from build123d import *

# Parameters (mm, degrees)
ESTRUSIONE_ESTRUSIONE1_DEPTH = 5
SCHIZZO2_W                   = 16
SCHIZZO2_H                   = 5
ESTRUSIONE_ESTRUSIONE2_DEPTH = 20
TAGLIO_ESTRUSIONE1_REACH     = 42.62
SCHIZZO3_R                   = 3.25


with BuildPart() as part:
    # Schizzo1 → Estrusione-Estrusione1 (new body)
    with BuildSketch(Plane.XY):
        Polygon((-16, 0), (0, 0), (0, -10), (20, -10), (20, -30), (4, -30), (-16, -9.295201316), align=None)
        with BuildLine():
            Line((16, -22.25), (6, -22.25))
            ThreePointArc((6, -22.25), (4.25, -24), (6, -25.75))
            Line((6, -25.75), (16, -25.75))
            ThreePointArc((16, -25.75), (17.75, -24), (16, -22.25))
        make_face(mode=Mode.SUBTRACT)
        with BuildLine():
            Line((16, -12.75), (6, -12.75))
            ThreePointArc((6, -12.75), (4.25, -14.5), (6, -16.25))
            Line((6, -16.25), (16, -16.25))
            ThreePointArc((16, -16.25), (17.75, -14.5), (16, -12.75))
        make_face(mode=Mode.SUBTRACT)
    extrude(amount=ESTRUSIONE_ESTRUSIONE1_DEPTH)

    # Schizzo2 → Estrusione-Estrusione2 (add)
    with BuildSketch(Plane.XY.offset(5)):
        with Locations((-8, -2.5)):
            Rectangle(SCHIZZO2_W, SCHIZZO2_H)
    extrude(amount=ESTRUSIONE_ESTRUSIONE2_DEPTH)

    # Schizzo3 → Taglio-Estrusione1 (cut, up to next)
    with BuildSketch(Plane.XZ.offset(5), mode=Mode.PRIVATE) as taglio_estrusione1_sk1:
        with Locations((-8, 17.5)):
            Circle(SCHIZZO3_R)
    taglio_estrusione1_tool1 = extrude(taglio_estrusione1_sk1.sketch, amount=-TAGLIO_ESTRUSIONE1_REACH, mode=Mode.PRIVATE) & part.part
    add(taglio_estrusione1_tool1.solids().sort_by_distance((-8, -5, 17.5))[0], mode=Mode.SUBTRACT)


solid = part.part
The model under review builds one solid part; all positions refer to its coordinate system, in mm. A direction names the side the tool comes from. Coordinates: 2 decimals unless noted, no trailing zeros. Write each loop counter-clockwise with the first axis right and the second up, starting at its lowest first coordinate (ties: lowest second). Pieces come first, ordered by that corner, then holes. Notation, with made-up numbers: (32, -23) -> (39, -23) arc R21 cw to (39, 12) -> close; hole circle Ø8 at (27.25, -23). An arc over 180 degrees is marked (long way). Answer in a Markdown table with one row per item.
1. For faces 1 (the flat face through (-8, -5, 13)), 2 (the flat face through (11, -22.25, 2)), 3 (the flat face through (12, -30, 2)), list the 3-axis set-ups (+Z, -Z, +X, -X, +Y, -Y) from which the entire face can be reached by the end or side of a thin tool; tool diameter is ignored.
Answers below:
| item | result |
|---|---|
| face 1 | +Z, +X, -X, -Y |
| face 2 | +Z, -Z |
| face 3 | +Z, -Z, +X, -X, -Y |
2. Clearance check with flat-ended pins moving along their axes: pin 1 Ø2.5 at (x, z) = (6, 3) entering from +Y; pin 2 Ø10 at (x, y) = (7.5, -22) entering from -Z; pin 3 Ø7.5 at (x, y) = (-6, -15) entering from +Z; pin 4 Ø13 at (x, z) = (-10.5, 19) entering from -Y. State where each tip first meets the part, or that it passes through.
Answers below:
| item | result |
|---|---|
| pin 1 | stops at y = -10 |
| pin 2 | stops at z = 0 |
| pin 3 | stops at z = 5 |
| pin 4 | stops at y = -5 |
3. Wall thickness on probe 1 along Z at (x, y) = (-8, -3.85); probe 2 along Z at (x, y) = (-10, -9); probe 3 along Y at (x, z) = (4, 3.75): over which ranges is each line inside the solid? List them lowest first. Write a range as [from, to].
Answers below:
| item | result |
|---|---|
| probe 1 | z = [0, 14.25], [20.75, 25] |
| probe 2 | z = [0, 5] |
| probe 3 | y = [-30, -10] |
4. We need section C-C, the plane y = -14.5. State the section outline as (x, z) points.
Answers below:
| item | result |
|---|---|
| outline | (-10.97, 0) -> (4.25, 0) -> (4.25, 5) -> (-10.97, 5) -> close; (17.75, 0) -> (20, 0) -> (20, 5) -> (17.75, 5) -> close |
5. Draft analysis for pull direction Y (two halves, no side actions). For faces 4 (the flat face through (10, -10, 2)), 5 (the flat face through (-16, -4, 10)), 6 (the cylindrical face through (4.25, -23.96, 2.46)), state which applies: +Y half, -Y half, draft (parallel to the pull), parting line (faces both ways), or undercut.
Answers below:
| item | result |
|---|---|
| face 4 | +Y half |
| face 5 | draft |
| face 6 | undercut |
6. We need section D-D, the plane x = 3. State the section outline as (y, z) points.
Answers below:
| item | result |
|---|---|
| outline | (-28.96, 0) -> (-10, 0) -> (-10, 5) -> (-28.96, 5) -> close |
7. We need section B-B, the plane x = 9.5. State the section outline as (y, z) points, and give its area (3 significant figures).
Answers below:
| item | result |
|---|---|
| outline | (-30, 0) -> (-25.75, 0) -> (-25.75, 5) -> (-30, 5) -> close; (-22.25, 0) -> (-16.25, 0) -> (-16.25, 5) -> (-22.25, 5) -> close; (-12.75, 0) -> (-10, 0) -> (-10, 5) -> (-12.75, 5) -> close |
| area | 65.0 mm^2 |
8. We need section A-A, the plane z = 17.5. State the section outline as (x, y) points.
Answers below:
| item | result |
|---|---|
| outline | (-16, -5) -> (-11.25, -5) -> (-11.25, 0) -> (-16, 0) -> close; (-4.75, -5) -> (0, -5) -> (0, 0) -> (-4.75, 0) -> close |
